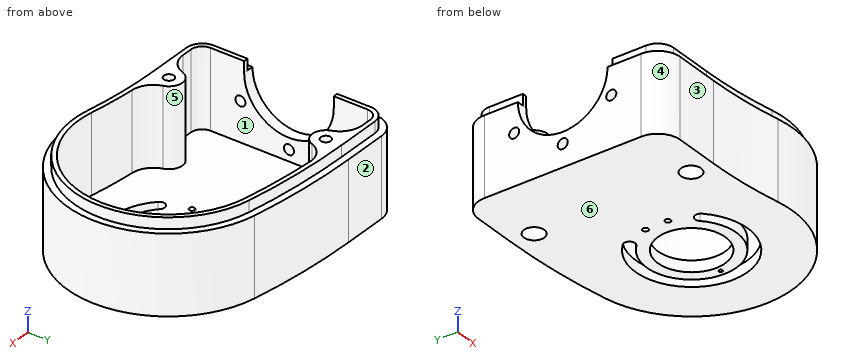
from build123d import *

# Parameters (mm, degrees)
EXTRUDE_1_DEPTH              = 35
CUT_EXTRUDE_1_DEPTH          = 30
SKETCH_3_R                   = 20
SKETCH_3_R_2                 = 2.25
CUT_EXTRUDE_2_DEPTH          = 10
SKETCH_4_R                   = 15
CUT_EXTRUDE_3_DEPTH          = 1
CUT_EXTRUDE_3_DEPTH_BACK     = 36
EXTRUDE_2_DEPTH              = 5
CUT_EXTRUDE_6_REACH          = 42
SKETCH_12_R                  = 6
EXTRUDE_3_DEPTH              = 35
FILLET_1_R                   = 10
HOLE_WIZARD_M2_1_D           = 1.6
HOLE_WIZARD_M2_1_DEPTH       = 5
HOLE_WIZARD_M3_1_D           = 2.5
HOLE_WIZARD_M3_1_DEPTH       = 5
HOLE_WIZARD_M4_6_D           = 4.5
HOLE_WIZARD_M4_6_DEPTH       = 40
HOLE_WIZARD_M4_6_CBORE_D     = 9
HOLE_WIZARD_M4_6_CBORE_DEPTH = 33.1
HOLE_WIZARD_M4_6_TIP         = 1.351936393


with BuildPart() as part:
    # 스케치1 → 보스-돌출1 (new body)
    with BuildSketch(Plane.XY):
        with BuildLine():
            Line((10, 45.518523903), (0, 45.518523903))
            Line((0, 45.518523903), (-10, 45.518523903))
            ThreePointArc((-10, 45.518523903), (-17.071067812, 42.589591715), (-20, 35.518523903))
            Line((-20, 35.518523903), (-20, -34.481476097))
            ThreePointArc((-20, -34.481476097), (-17.071067812, -41.552543909), (-10, -44.481476097))
            Line((-10, -44.481476097), (0, -44.481476097))
            Line((0, -44.481476097), (10, -44.481476097))
            ThreePointArc((10, -44.481476097), (27.43114855, -45.242536479), (44.729635533, -47.519925495))
            ThreePointArc((44.729635533, -47.519925495), (96.860152414, -11.017744604), (60.357971523, 41.112772276))
            ThreePointArc((60.357971523, 41.112772276), (35.275165397, 44.414986349), (10, 45.518523903))
        make_face()
    extrude(amount=EXTRUDE_1_DEPTH)

    # 스케치2 → 컷-돌출1 (cut)
    with BuildSketch(Plane.XY.offset(35)):
        with BuildLine():
            Line((10, 40.518523903), (-10, 40.518523903))
            ThreePointArc((-10, 40.518523903), (-13.535533906, 39.054057809), (-15, 35.518523903))
            Line((-15, 35.518523903), (-15, -34.481476097))
            ThreePointArc((-15, -34.481476097), (-13.535533906, -38.017010003), (-10, -39.481476097))
            Line((-10, -39.481476097), (10, -39.481476097))
            ThreePointArc((10, -39.481476097), (27.866927263, -40.261562989), (45.597876422, -42.59588673))
            ThreePointArc((45.597876422, -42.59588673), (91.936113649, -10.149503716), (59.489730635, 36.188733511))
            ThreePointArc((59.489730635, 36.188733511), (34.839386683, 39.434012859), (10, 40.518523903))
        make_face()
    extrude(amount=-CUT_EXTRUDE_1_DEPTH, mode=Mode.SUBTRACT)

    # 스케치3 → 컷-돌출2 (cut)
    with BuildSketch(Plane.ZY.offset(20)):
        with Locations((35, 0.518523903)):
            Circle(SKETCH_3_R)
        with Locations((22.5, 22.169158997)):
            Circle(SKETCH_3_R_2)
        with Locations((10, 0.518523903)):
            Circle(SKETCH_3_R_2)
        with Locations((22.5, -21.132111192)):
            Circle(SKETCH_3_R_2)
    extrude(amount=-CUT_EXTRUDE_2_DEPTH, mode=Mode.SUBTRACT)

    # 스케치4 → 컷-돌출3 (cut, two sides)
    with BuildSketch(Plane(origin=(0, 0, 0), x_dir=(-1, 0, 0), z_dir=(0, 0, -1))) as cut_extrude_3_sk:
        with Locations((-52.543803528, -3.203576609)):
            Circle(SKETCH_4_R)
    extrude(amount=CUT_EXTRUDE_3_DEPTH, mode=Mode.SUBTRACT)
    extrude(cut_extrude_3_sk.sketch, amount=-CUT_EXTRUDE_3_DEPTH_BACK, mode=Mode.SUBTRACT)

    # 스케치8 → 보스-돌출2 (add)
    with BuildSketch(Plane.XY.offset(35)):
        with BuildLine():
            Line((-15, -19.481476097), (-15, -34.481476097))
            ThreePointArc((-15, -34.481476097), (-13.535533906, -38.017010003), (-10, -39.481476097))
            Line((-10, -39.481476097), (10, -39.481476097))
            ThreePointArc((10, -39.481476097), (27.866927263, -40.261562989), (45.597876422, -42.59588673))
            ThreePointArc((45.597876422, -42.59588673), (91.936113649, -10.149503716), (59.489730635, 36.188733511))
            ThreePointArc((59.489730635, 36.188733511), (34.839386683, 39.434012859), (10, 40.518523903))
            Line((10, 40.518523903), (-10, 40.518523903))
            ThreePointArc((-10, 40.518523903), (-13.535533906, 39.054057809), (-15, 35.518523903))
            Line((-15, 35.518523903), (-15, 20.518523903))
            Line((-15, 20.518523903), (-17, 20.518523903))
            Line((-17, 20.518523903), (-17, 35.518523903))
            ThreePointArc((-17, 35.518523903), (-14.949747468, 40.468271371), (-10, 42.518523903))
            Line((-10, 42.518523903), (10, 42.518523903))
            ThreePointArc((10, 42.518523903), (35.013698169, 41.426402255), (59.83702699, 38.158349017))
            ThreePointArc((59.83702699, 38.158349017), (93.905729155, -10.496800071), (45.250580066, -44.565502236))
            ThreePointArc((45.250580066, -44.565502236), (27.692615778, -42.253952385), (10, -41.481476097))
            Line((10, -41.481476097), (-10, -41.481476097))
            ThreePointArc((-10, -41.481476097), (-14.949747468, -39.431223566), (-17, -34.481476097))
            Line((-17, -34.481476097), (-17, -19.481476097))
            Line((-17, -19.481476097), (-15, -19.481476097))
        make_face()
    extrude(amount=EXTRUDE_2_DEPTH)

    # 스케치9 → 컷-돌출6 (cut, up to next)
    with BuildSketch(Plane(origin=(0, 0, 0), x_dir=(-1, 0, 0), z_dir=(0, 0, -1)), mode=Mode.PRIVATE) as cut_extrude_6_sk1:
        with BuildLine():
            ThreePointArc((-38.401667905, 10.938559014), (-34.866133999, 10.938559014), (-34.866133999, 14.47409292))
            ThreePointArc((-34.866133999, 14.47409292), (-77.543803528, -3.203576609), (-34.866133999, -20.881246139))
            ThreePointArc((-34.866133999, -20.881246139), (-34.866133999, -17.345712233), (-38.401667905, -17.345712233))
            ThreePointArc((-38.401667905, -17.345712233), (-72.543803528, -3.203576609), (-38.401667905, 10.938559014))
        make_face()
    cut_extrude_6_tool1 = extrude(cut_extrude_6_sk1.sketch, amount=-CUT_EXTRUDE_6_REACH, mode=Mode.PRIVATE) & part.part
    add(cut_extrude_6_tool1.solids().sort_by_distance((35.334344, -17.813923, 0))[0], mode=Mode.SUBTRACT)

    # 스케치12 → 보스-돌출3 (add)
    with BuildSketch(Plane.XY.offset(5)):
        with Locations((10, 35.518523903)):
            Circle(SKETCH_12_R)
        with Locations((10, -34.481476097)):
            Circle(SKETCH_12_R)
    extrude(amount=EXTRUDE_3_DEPTH)

    # 필렛1
    fillet_1_edges = [part.edges().sort_by_distance(p)[0] for p in [
        (13.346048824, 40.498881046, 22.5),
        (6.68337521, 40.518523903, 22.5),
        (13.276798635, -39.507666574, 22.5),
        (6.68337521, -39.481476097, 22.5),
    ]]
    fillet(fillet_1_edges, radius=FILLET_1_R)

    # M2 나사 구멍1
    with Locations(Plane.XY.offset(5)):
        with Locations((70.043803528, -3.203576609)):
            Hole(HOLE_WIZARD_M2_1_D / 2, depth=HOLE_WIZARD_M2_1_DEPTH)

    # M3 나사 구멍1
    with Locations(Plane.XY.offset(5)):
        with Locations((31.543803528, 1.796423391), (31.543803528, -8.203576609)):
            Hole(HOLE_WIZARD_M3_1_D / 2, depth=HOLE_WIZARD_M3_1_DEPTH)

    # M4 남비 머리 나사용 카운터보어6
    with Locations(Plane(origin=(0, 0, 0), x_dir=(-1, 0, 0), z_dir=(0, 0, -1))):
        with Locations((-10, 35.518523903), (-10, -34.481476097)):
            CounterBoreHole(HOLE_WIZARD_M4_6_D / 2, HOLE_WIZARD_M4_6_CBORE_D / 2, HOLE_WIZARD_M4_6_CBORE_DEPTH, depth=HOLE_WIZARD_M4_6_DEPTH)
            with Locations((0, 0, -(HOLE_WIZARD_M4_6_DEPTH + HOLE_WIZARD_M4_6_TIP / 2))):  # 118° drill point
                Cone(0, HOLE_WIZARD_M4_6_D / 2, HOLE_WIZARD_M4_6_TIP, mode=Mode.SUBTRACT)


solid = part.part
Work out the finished part from the listing and answer in its coordinate system (mm). Face numbers are marked on the shaded views. A direction names the side the tool comes from. Give positions to 0.01 mm unless a question says otherwise; leave off trailing zeros. Order: outer loops, then holes, each group sorted by start corner. A loop starts at its lowest first (then second) coordinate and runs counter-clockwise, first axis right, second up. Notation, with made-up numbers: M 6.5,-15 L 17.5,-15 A27 cw 17.5,12 Z; hole C 70,22 d5. An arc over 180 degrees is marked long. Return JSON: item names as keys, results as strings.
Q1. Which of the six approach directions +Z, -Z, +X, -X, +Y, -Y give full straight-line access (tool end or side, diameter ignored) to the marked faces 1, 2 and 3?
Answer below:
{"face 1": "+Z", "face 2": "+Z, -Z, +X, -X, +Y", "face 3": "+Z, -Z, -X, -Y"}
Q2. The mould has two halves that part along Y. Classify the marked faces 4, 5 and 6: pulls with the +Y half, pulls with the -Y half, needs draft (parallel to the pull), parting line crosses it, or undercut.
Answer below:
{"face 4": "pulls with the -Y half", "face 5": "undercut", "face 6": "needs draft"}
Q3. Each of these flat-tipped pins is pushed along its axis until it touches: pin 1 (10 mm diameter, centred on x = 10.5, y = -36, fed in from -Z); pin 2 (2.5 mm diameter, centred on y = 28, z = 37, fed in from -X); pin 3 (2 mm diameter, centred on x = 31.54, y = -8.2, fed in from -Z); pin 4 (5 mm diameter, centred on y = -8, z = 9.5, fed in from +X). Where does it stop, or does it pass through?
Answer below:
{"pin 1": "stops at z = 0", "pin 2": "stops at x = -17", "pin 3": "passes through", "pin 4": "stops at x = 97.49"}
Q4. Find the intervals of material crossed by line 1 along Y through (x, z) = (10, 19); line 2 along Y through (x, z) = (10, 36); line 3 along X through (y, z) = (-4.5, 12), in increasing order. Write a range as [from, to].
Answer below:
{"line 1": "y = [-44.48, -38.98], [-29.98, -28.48], [29.52, 31.02], [40.02, 45.52]", "line 2": "y = [-41.48, -36.73], [-32.23, -28.48], [29.52, 33.27], [37.77, 42.52]", "line 3": "x = [-20, -15], [92.52, 97.53]"}
Q5. Find section A-A, the plane z = 13.5. State how many separate pieces and enclosed holes the cut face has, and give its area (3 significant figures).
Answer below:
{"separate pieces": "1", "enclosed holes": "3", "area": "1,930 mm^2"}
Q6. Find section C-C, the plane y = 26. Write down the section's boundary in (x, z), and give its area (3 significant figures).
Answer below:
{"outline": "M -20,0 L 86.78,0 L 86.78,35 L 82.73,35 L 82.73,40 L 79.88,40 L 79.88,5 L -15,5 L -15,40 L -17,40 L -17,35 L -20,35 Z", "area": "915 mm^2"}
